from build123d import *

# Parameters (mm, degrees)
F0_R     = 28.1638511083
F1_DEPTH = 35


# Not quite as in the source:
# - the program builds the solid bodies; features that only make, move or delete a surface that nothing else refers to are left out


with BuildPart() as f1:
    # F0 (on Front) → F1 (new body)
    with BuildSketch(Plane.XZ):
        with BuildLine():
            ThreePointArc((10.057095516, 52.6112248036), (41.2782201188, 34.1349482111), (53.5638511083, 0))
            ThreePointArc((53.5638511083, 0), (41.2782201188, -34.1349482111), (10.057095516, -52.6112248036))
            Line((10.057095516, -52.6112248036), (154.7690787877, -24.9482642185))
            ThreePointArc((154.7690787877, -24.9482642185), (124.6, 0), (154.7690787877, 24.9482642185))
            Line((154.7690787877, 24.9482642185), (10.057095516, 52.6112248036))
        make_face()
        with BuildLine():
            ThreePointArc((10.057095516, -52.6112248036), (41.2782201188, -34.1349482111), (53.5638511083, 0))
            ThreePointArc((53.5638511083, 0), (41.2782201188, 34.1349482111), (10.057095516, 52.6112248036))
            ThreePointArc((10.057095516, 52.6112248036), (-53.5638511083, 0), (10.057095516, -52.6112248036))
        make_face()
        Circle(F0_R, mode=Mode.SUBTRACT)
        with BuildLine():
            ThreePointArc((175.4, 0), (169.5741487836, 16.1868063372), (154.7690787877, 24.9482642185))
            ThreePointArc((154.7690787877, 24.9482642185), (124.6, 0), (154.7690787877, -24.9482642185))
            ThreePointArc((154.7690787877, -24.9482642185), (169.5741487836, -16.1868063372), (175.4, 0))
        make_face()
    extrude(amount=F1_DEPTH)


solid = f1.part
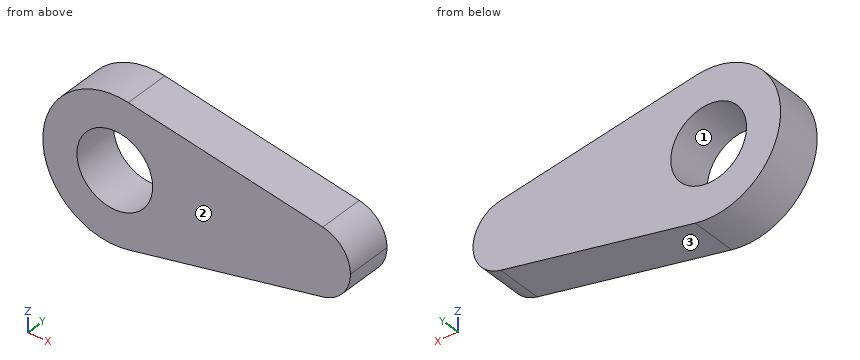
Geometry: final body of the model. Coordinates: model frame, mm. Face numbers are marked on the shaded views. Round coordinates to 2 decimals unless told otherwise and drop trailing zeros. Loops run counter-clockwise (first coordinate to the right, second up) from the corner with the lowest first, then second, coordinate; pieces in that order, holes last.
Q1. Section A-A on x = 0. Return loops of the section in (y, z), plus the area to 3 significant figures.
Q2. Pull-direction query (X, two-part tool) for the marked faces 1, 2 and 3; classes: released by +X, released by -X, zero draft, split by the parting line, or undercut.
Q3. Section D-D on x = 112. Return loops of the section in (y, z), plus the area to 3 significant figures.
Q4. Section C-C on z = -13. Return loops of the section in (x, y), plus the area to 3 significant figures.
Q5. Material intervals for L1, parallel to Z at x = 0, y = -12; L2, parallel to X at y = -20, z = 16; L3, parallel to Z at x = 12, y = -28, sorted ascending.
Q6. Pin query (flat end, axial travel): P1, Ø4, axis at x = 137, y = -29.5, coming from the -Z side; P2, Ø1.5, axis at x = 42, y = -5, coming from the -Z side; P3, Ø6, axis at y = -17.5, z = 20.5, coming from the +X side. Return the tip coordinate at first contact, or that it passes through.
Q7. Section B-B on y = -9.5. Return loops of the section in (x, z).
Evaluation:
1. outline: (-35, -53.56) - (0, -53.56) - (0, -28.16) - (-35, -28.16) - close; (-35, 28.16) - (0, 28.16) - (0, 53.56) - (-35, 53.56) - close
1. area: 1,780 mm2
2. face 1: undercut
2. face 2: zero draft
2. face 3: released by +X
3. outline: (-35, -33.12) - (0, -33.12) - (0, 33.12) - (-35, 33.12) - close
3. area: 2,320 mm2
4. outline: (-51.96, -35) - (-24.98, -35) - (-24.98, 0) - (-51.96, 0) - close; (24.98, -35) - (171.82, -35) - (171.82, 0) - (24.98, 0) - close
4. area: 6,080 mm2
5. L1: z = -53.56 to -28.16, 28.16 to 53.56
5. L2: x = -51.12 to -23.18, 23.18 to 169.73
5. L3: z = -52.24 to -25.48, 25.48 to 52.24
6. P1: stops at z = -28.73
6. P2: stops at z = -46.65
6. P3: stops at x = 168.41
7. outline: (10.06, -52.61) - (154.77, -24.95) arc R25.4 ccw to (154.77, 24.95) - (10.06, 52.61) arc R53.56 ccw (long way) to start; hole circle Ø56.33 at (0, 0)
